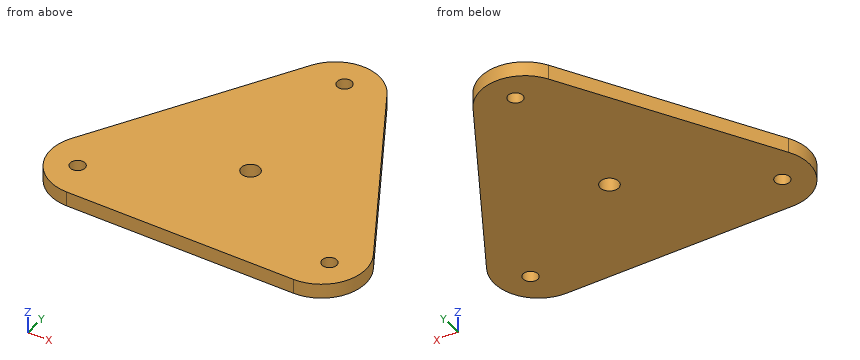
Autodesk Inventor part; units mm, degrees
ref_plane "YZ Plane" through (0, 0, 0) normal (1, 0, 0) x (0, 1, 0)
ref_plane "XZ Plane" through (0, 0, 0) normal (0, 1, 0) x (-1, 0, 0)
ref_plane "XY Plane" through (0, 0, 0) normal (0, 0, 1) x (1, 0, 0)
sketch "Sketch2" plane through (0, 0, 0) normal (0, 0, 1) x (1, 0, 0)
  circle A0 centre (0, 0) radius 3.9688
  circle A1 centre (0, 63.5) radius 3.175
  circle A2 centre (-54.9926, -31.75) radius 3.175
  circle A3 centre (54.9926, -31.75) radius 3.175
  line L0 (0, 69.85) -> (60.4919, -34.925) construction
  line L1 (60.4919, -34.925) -> (-60.4919, -34.925) construction
  line L2 (-60.4919, -34.925) -> (0, 69.85) construction
  line L3 (0, 95.25) -> (82.4889, -47.625)
  line L4 (82.4889, -47.625) -> (-82.4889, -47.625)
  line L5 (-82.4889, -47.625) -> (0, 95.25)
  dimension "d0" = 7.9375
  dimension "d1" = 6.35
  dimension "d2" = 63.5
  dimension "d5" = 360
  dimension "d8" = 12.7
  dimension "d9" = 12.7
  dimension "d10" = 12.7
extrude "Extrusion1" add sketch "Sketch2" along normal blind 6.35
fillet "Fillet1" radius 19.05 3 edges at (0, 95.25, 3.175) (-82.4889, -47.625, 3.175) (82.4889, -47.625, 3.175)
properties part number "Triangle-5-16-hole"
Here's how the part is built. I have some questions about the finished solid (model axes, mm). Give positions to 0.01 mm unless a question says otherwise; leave off trailing zeros. Write each loop counter-clockwise with the first axis right and the second up, starting at its lowest first coordinate (ties: lowest second). Pieces come first, ordered by that corner, then holes. Notation, with made-up numbers: (-23, 54.5) -> (31, 54.5) arc R26 cw to (31, 91.5) -> close; hole circle Ø6 at (78.25, 84). An arc over 180 degrees is marked (long way). Use one line per item in the form item = value. Start each with the question number.
1. Imagine slicing it at C-C on x = 0. List the corners of the cut face in (y, z) for me (3 decimals), plus the area to 3 significant figures.
2. Imagine slicing it at D-D on y = -31.75. List the corners of the cut face in (x, z) for me.
3. Will these pins go through, and if not, where does the flat tip stop? pin 1 Ø3 at (y, z) = (55.5, 4) entering from +X; pin 2 Ø3 at (y, z) = (18, 5.5) entering from +X.
4. If I drill on L1, parallel to Y at x = 0, z = 3 (3 decimals); L2, parallel to X at y = 3.5, z = 3.5; L3, parallel to Y at x = 31, z = 6.25 (3 decimals), over which ranges is the centre line in solid material (lowest first)?
5. Imagine slicing it at A-A on z = 1.5. List the corners of the cut face in (x, y) for me (3 decimals), plus the area to 3 significant figures.
6. Imagine slicing it at B-B on y = 0. List the corners of the cut face in (x, z) for me, plus the area to 3 significant figures.
Entries:
q1.outline = (-47.625, 0) -> (-3.969, 0) -> (-3.969, 6.35) -> (-47.625, 6.35) -> close; (3.969, 0) -> (60.325, 0) -> (60.325, 6.35) -> (3.969, 6.35) -> close; (66.675, 0) -> (76.2, 0) -> (76.2, 6.35) -> (66.675, 6.35) -> close
q1.area = 696 mm²
q2.outline = (-68.28, 0) -> (-58.17, 0) -> (-58.17, 6.35) -> (-68.28, 6.35) -> close; (-51.82, 0) -> (51.82, 0) -> (51.82, 6.35) -> (-51.82, 6.35) -> close; (58.17, 0) -> (68.28, 0) -> (68.28, 6.35) -> (58.17, 6.35) -> close
q3.pin_1 = 23.82
q3.pin_2 = 45.47
q4.L1 = -47.625 to -3.969, 3.969 to 60.325, 66.675 to 76.2
q4.L2 = -52.97 to -1.87, 1.87 to 52.97
q4.L3 = -47.625 to 41.556
q5.outline = (-65.991, -19.05) arc R19.05 ccw to (-49.493, -47.625) -> (49.493, -47.625) arc R19.05 ccw to (65.991, -19.05) -> (16.498, 66.675) arc R19.05 ccw to (-16.498, 66.675) -> close; hole circle Ø6.35 at (-54.993, -31.75); hole circle Ø7.938 at (0, 0); hole circle Ø6.35 at (0, 63.5); hole circle Ø6.35 at (54.993, -31.75)
q5.area = 10,900 mm²
q6.outline = (-54.99, 0) -> (-3.97, 0) -> (-3.97, 6.35) -> (-54.99, 6.35) -> close; (3.97, 0) -> (54.99, 0) -> (54.99, 6.35) -> (3.97, 6.35) -> close
q6.area = 648 mm²
